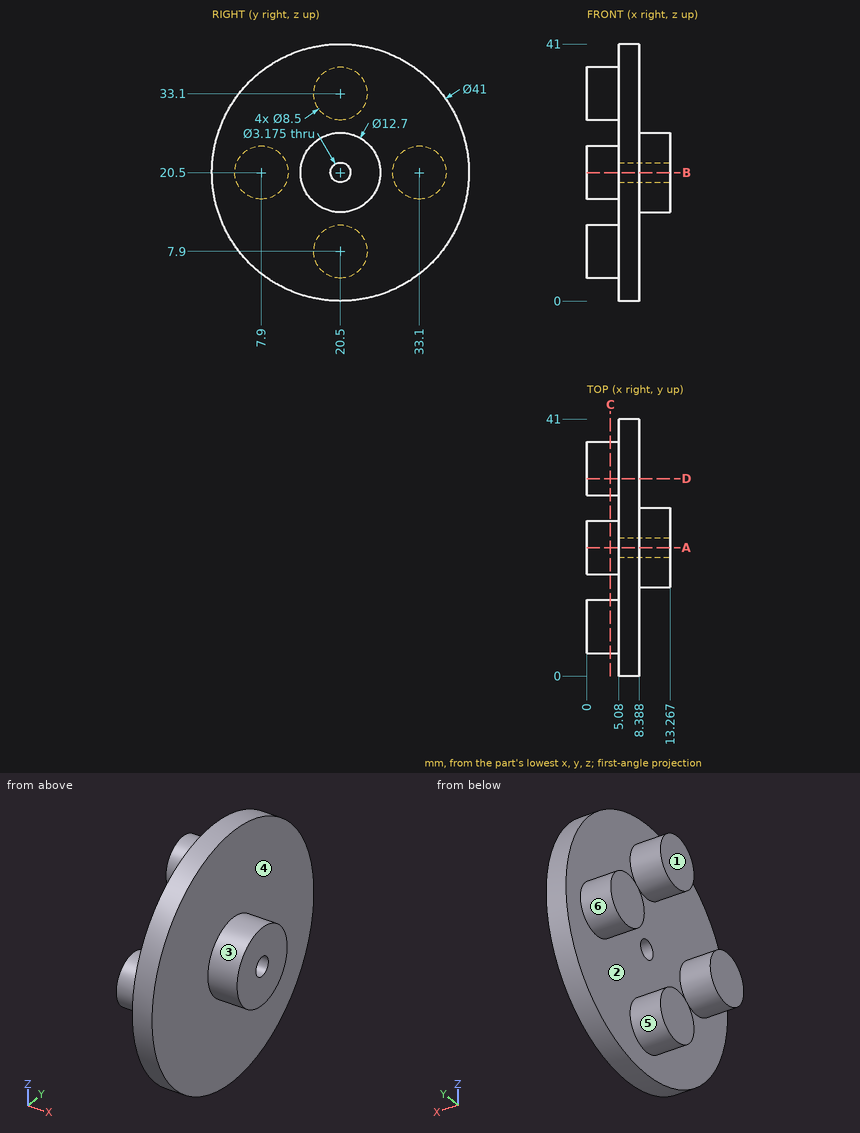
Geometry check sheet. Reference: drawing and pictorial views, mm from the part's lowest x, y, z. A direction names the side the tool comes from. Give positions to 0.01 mm unless a question says otherwise; leave off trailing zeros. Loops run counter-clockwise (first coordinate to the right, second up) from the corner with the lowest first, then second, coordinate; pieces in that order, holes last. Notation, with made-up numbers: (34, 57) -> (84, 57) arc R17 ccw to (84, 80) -> close; hole circle Ø6 at (-9.75, -38.75). An arc over 180 degrees is marked (long way). Answer in a Markdown table with one row per item. Add a question column.
1) Gauge pin test, flat ends, axial feed: P1, Ø1, axis at x = 11, y = 24.5, coming from the -Z side; P2, Ø2.5, axis at y = 20.5, z = 20.5, coming from the -X side; P3, Ø1, axis at x = 7.5, z = 14, coming from the +Y side; P4, Ø2, axis at y = 9, z = 35.5, coming from the -X side. Record the tip position at first contact, or that the pin passes through.
2) Cross-section at A-A on y = 20.5. Record the boundary of the cut face in (x, z).
3) Draft check along Z on the marked faces 4, 5 and 6. Enter one of: pulls with the +Z half, pulls with the -Z half, needs draft (parallel to the pull), parting line crosses it, or undercut.
4) Cross-section at C-C on x = 3.75. Record the boundary of the cut face in (y, z), and give its area (3 significant figures).
5) Set-up check for the marked faces 1, 2 and 3: record each of +Z, -Z, +X, -X, +Y, -Y from which the full face is reachable in a straight line by a thin tool's end or side.
6) Cross-section at D-D on y = 31.5. Record the boundary of the cut face in (x, z).
7) Material ranges on probe 1 along Y at (x, z) = (10, 20.5); probe 2 along Y at (x, z) = (7, 20.5), recorded low to high. Write a range as from..to.
Outcome:
| question | item | result |
|---|---|---|
| 1 | P1 | stops at z = 15.2 |
| 1 | P2 | passes through |
| 1 | P3 | stops at y = 40.1 |
| 1 | P4 | stops at x = 5.08 |
| 2 | outline | (0, 3.65) -> (5.08, 3.65) -> (5.08, 0) -> (8.39, 0) -> (8.39, 14.15) -> (13.27, 14.15) -> (13.27, 18.91) -> (5.08, 18.91) -> (5.08, 12.15) -> (0, 12.15) -> close; (0, 28.85) -> (5.08, 28.85) -> (5.08, 22.09) -> (13.27, 22.09) -> (13.27, 26.85) -> (8.39, 26.85) -> (8.39, 41) -> (5.08, 41) -> (5.08, 37.35) -> (0, 37.35) -> close |
| 3 | face 4 | needs draft |
| 3 | face 5 | undercut |
| 3 | face 6 | parting line crosses it |
| 4 | outline | circle Ø8.5 at (7.9, 20.5); circle Ø8.5 at (20.5, 7.9); circle Ø8.5 at (20.5, 33.1); circle Ø8.5 at (33.1, 20.5) |
| 4 | area | 227 mm^2 |
| 5 | face 1 | +Z, -Z, -X, +Y, -Y |
| 5 | face 2 | -X |
| 5 | face 3 | +X |
| 6 | outline | (0, 16.56) -> (5.08, 16.56) -> (5.08, 3.2) -> (8.39, 3.2) -> (8.39, 37.8) -> (5.08, 37.8) -> (5.08, 24.44) -> (0, 24.44) -> close |
| 7 | probe 1 | y = 14.15..18.91, 22.09..26.85 |
| 7 | probe 2 | y = 0..18.91, 22.09..41 |
